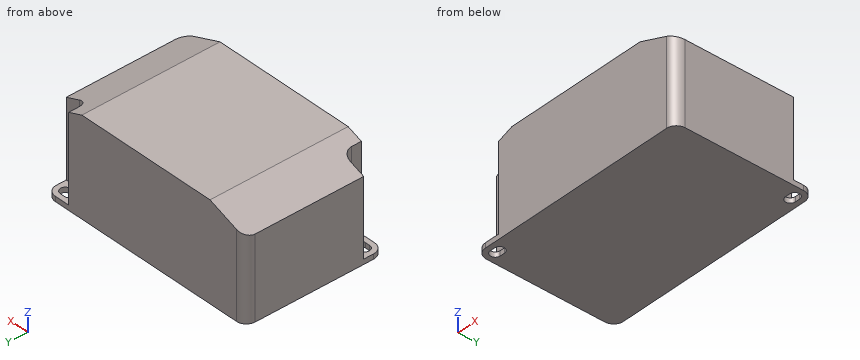
from build123d import *

# Parameters (mm, degrees)
F0_W        = 5
F0_H        = 4
F1_DEPTH    = 19.5
F2_T1_DEPTH = 69.5019292892
F3_START    = 1
F3_DEPTH    = 24
F4_R        = 2


# Not quite as in the source:
# - a fillet or chamfer that OpenCascade refuses, or shapes differently, is made with other operations: its cross-section is extruded or revolved along the edge and cut away or added


with BuildPart() as f1:
    # F0 (on Top) → F1 (new body)
    with BuildSketch(Plane.XY):
        Polygon((17.5, 14), (-22.5, 14), (-22.5, -10), (-17.5, -10), (-17.5, -14), (22.5, -14), (22.5, 10), (17.5, 10), align=None)
        with Locations((20, 12)):
            Rectangle(F0_W, F0_H)
        with BuildLine():
            ThreePointArc((19.5, 11), (18.5, 12), (19.5, 13))
            Line((19.5, 13), (20.5, 13))
            ThreePointArc((20.5, 13), (21.5, 12), (20.5, 11))
            Line((20.5, 11), (19.5, 11))
        make_face(mode=Mode.SUBTRACT)
        with Locations((-20, -12)):
            Rectangle(F0_W, F0_H)
        with BuildLine():
            ThreePointArc((-20.5, -13), (-21.5, -12), (-20.5, -11))
            Line((-20.5, -11), (-19.5, -11))
            ThreePointArc((-19.5, -11), (-18.5, -12), (-19.5, -13))
            Line((-19.5, -13), (-20.5, -13))
        make_face(mode=Mode.SUBTRACT)
    extrude(amount=F1_DEPTH)

    # F2: chamfer of 3 x 8 on 2 edges, made by hand

    # F2_s2 → F2_t1 (cut)
    with BuildSketch(Plane.XZ.offset(-34.7509646446)):
        Polygon((-22.5, 16.5), (-14.5, 19.5), (-22.5, 19.5), align=None)
        Polygon((22.5, 16.5), (14.5, 19.5), (22.5, 19.5), align=None)
    extrude(amount=F2_T1_DEPTH, mode=Mode.SUBTRACT)

    # F0 (on Top) → F3 (cut)
    with BuildSketch(Plane.XY.offset(F3_START)):
        with Locations((-20, -12)):
            Rectangle(F0_W, F0_H)
        with BuildLine():
            ThreePointArc((-20.5, -13), (-21.5, -12), (-20.5, -11))
            Line((-20.5, -11), (-19.5, -11))
            ThreePointArc((-19.5, -11), (-18.5, -12), (-19.5, -13))
            Line((-19.5, -13), (-20.5, -13))
        make_face(mode=Mode.SUBTRACT)
        with Locations((20, 12)):
            Rectangle(F0_W, F0_H)
        with BuildLine():
            ThreePointArc((19.5, 11), (18.5, 12), (19.5, 13))
            Line((19.5, 13), (20.5, 13))
            ThreePointArc((20.5, 13), (21.5, 12), (20.5, 11))
            Line((20.5, 11), (19.5, 11))
        make_face(mode=Mode.SUBTRACT)
    extrude(amount=F3_DEPTH, mode=Mode.SUBTRACT)

    # F4
    f4_edges = [f1.edges().sort_by_distance(p)[0] for p in [
        (-17.5, -10, 9.6875),
        (17.5, 10, 9.6875),
        (22.5, -14, 8.25),
        (22.5, 14, 0.5),
        (-22.5, 14, 8.25),
        (-22.5, -14, 0.5),
    ]]
    fillet(f4_edges, radius=F4_R)


solid = f1.part
Can you work these out from the model? Positions are in its coordinate system, mm. Give positions to 0.01 mm unless a question says otherwise; leave off trailing zeros. Write each loop counter-clockwise with the first axis right and the second up, starting at its lowest first coordinate (ties: lowest second). Pieces come first, ordered by that corner, then holes. Notation, with made-up numbers: M -25,-9 L -21,-9 A25 ccw -21,6 Z; hole C 15.5,-21.75 d7. An arc over 180 degrees is marked long. Answer in a Markdown table with one row per item. Add a question column.
Item 1: Imagine slicing it at C-C, the plane x = -16.5. Write out the boundary of the cut face in (y, z).
Item 2: Please list where these lines run through material, in increasing order: L1, parallel to X at y = 10.25, z = 13; L2, parallel to Z at x = 18, y = 4.5; L3, parallel to Z at x = -20, y = 10.
Item 3: For pin 1 Ø2.5 at (x, z) = (20.5, 8.5) entering from +Y; pin 2 Ø10 at (x, y) = (18, -2) entering from +Z; pin 3 Ø0.6 at (y, z) = (-13.5, 6.5) entering from -X; pin 4 Ø0.6 at (y, z) = (13, 13) entering from +X, each with a flat end and sliding along its axis, tell me the tip position at first contact or that it passes through.
Item 4: Imagine slicing it at A-A, the plane z = 9. Write out the boundary of the cut face in (x, y), plus the area to 3 significant figures.
Item 5: Imagine slicing it at B-B, the plane y = -5.5. Write out the boundary of the cut face in (x, z), plus the area to 4 significant figures.
Evaluation:
| question | item | result |
|---|---|---|
| 1 | outline | M -14,0 L 14,0 L 14,18.75 L -14,18.75 Z |
| 2 | L1 | x = -22.5 to 18.53 |
| 2 | L2 | z = 0 to 18.19 |
| 2 | L3 | z = 0 to 17.44 |
| 3 | pin 1 | stops at y = 10.02 |
| 3 | pin 2 | stops at z = 19.5 |
| 3 | pin 3 | stops at x = -17.5 |
| 3 | pin 4 | stops at x = 17.5 |
| 4 | outline | M -22.5,-10 L -19.5,-10 A2 cw -17.5,-12 L -17.5,-14 L 20.5,-14 A2 ccw 22.5,-12 L 22.5,10 L 19.5,10 A2 cw 17.5,12 L 17.5,14 L -20.5,14 A2 ccw -22.5,12 Z |
| 4 | area | 1,220 mm² |
| 5 | outline | M -22.5,0 L 22.5,0 L 22.5,16.5 L 14.5,19.5 L -14.5,19.5 L -22.5,16.5 Z |
| 5 | area | 853.5 mm² |
